```python
from build123d import *

# Parameters (mm, degrees)
SKETCH_1_R          = 2
SKETCH_1_W          = 8.7
SKETCH_1_H          = 18
EXTRUDE_1_DEPTH     = 5
FILLET_1_R          = 2
CUT_EXTRUDE_1_REACH = 58.089


with BuildPart() as part:
    # Sketch 1 → Extrude 1 (new body)
    # profile 1 of 3: a face of its own
    with BuildSketch(Plane.XY):
        with BuildLine():
            Line((39, 40), (-39, 40))
            Line((-39, 40), (-39, 0))
            Line((-39, 0), (-30.3, 0))
            ThreePointArc((-30.3, 0), (0, 30.3), (30.3, 0))
            Line((30.3, 0), (39, 0))
            Line((39, 0), (39, 40))
        make_face()
        with Locations((-34.65, 10)):
            Circle(SKETCH_1_R, mode=Mode.SUBTRACT)
        with Locations((34.65, 10)):
            Circle(SKETCH_1_R, mode=Mode.SUBTRACT)
    # profile 2 of 3: a face of its own
    with BuildSketch(Plane.XY):
        with Locations((-34.65, -9)):
            Rectangle(SKETCH_1_W, SKETCH_1_H)
        with Locations((-34.65, -10)):
            Circle(SKETCH_1_R, mode=Mode.SUBTRACT)
    # profile 3 of 3: a face of its own
    with BuildSketch(Plane.XY):
        with Locations((34.65, -9)):
            Rectangle(SKETCH_1_W, SKETCH_1_H)
        with Locations((34.65, -10)):
            Circle(SKETCH_1_R, mode=Mode.SUBTRACT)
    extrude(amount=EXTRUDE_1_DEPTH)

    # Fillet 1
    fillet_1_edges = [part.edges().sort_by_distance(p)[0] for p in [
        (-30.3, -18, 2.5),
        (-39, -18, 2.5),
        (-39, 40, 2.5),
        (39, 40, 2.5),
        (39, -18, 2.5),
        (30.3, -18, 2.5),
    ]]
    fillet(fillet_1_edges, radius=FILLET_1_R)

    # Sketch 2 → Cut-Extrude 1 (cut, up to next)
    with BuildSketch(Plane.XY.offset(5), mode=Mode.PRIVATE) as cut_extrude_1_sk1:
        with BuildLine():
            Line((-36.65, 10), (-36.65, 12))
            ThreePointArc((-36.65, 12), (-34.65, 14), (-32.65, 12))
            Line((-32.65, 12), (-32.65, 10))
            Line((-32.65, 10), (-36.65, 10))
        make_face()
    cut_extrude_1_tool1 = extrude(cut_extrude_1_sk1.sketch, amount=-CUT_EXTRUDE_1_REACH, mode=Mode.PRIVATE) & part.part
    # Sketch 2 → Cut-Extrude 1 (cut, up to next)
    with BuildSketch(Plane.XY.offset(5), mode=Mode.PRIVATE) as cut_extrude_1_sk2:
        with BuildLine():
            Line((-36.65, -10), (-36.65, -8))
            ThreePointArc((-36.65, -8), (-34.65, -6), (-32.65, -8))
            Line((-32.65, -8), (-32.65, -10))
            Line((-32.65, -10), (-36.65, -10))
        make_face()
    cut_extrude_1_tool2 = extrude(cut_extrude_1_sk2.sketch, amount=-CUT_EXTRUDE_1_REACH, mode=Mode.PRIVATE) & part.part
    cut_extrude_1_1 = cut_extrude_1_tool1.solids().sort_by_distance((-34.65, 11.8133, 5))[0]
    add(cut_extrude_1_1, mode=Mode.SUBTRACT)
    cut_extrude_1_2 = cut_extrude_1_tool2.solids().sort_by_distance((-34.65, -8.1867, 5))[0]
    add(cut_extrude_1_2, mode=Mode.SUBTRACT)
    cut_extrude_1 = cut_extrude_1_1 + cut_extrude_1_2  # Cut-Extrude 1 as one shape, for the pattern or mirror that repeats it

    # Mirror 1: Cut-Extrude 1 across plane
    add(cut_extrude_1.mirror(Plane(origin=(0, 0, 0), x_dir=(0, 0, 1), z_dir=(1, 0, 0))), mode=Mode.SUBTRACT)


solid = part.part
```
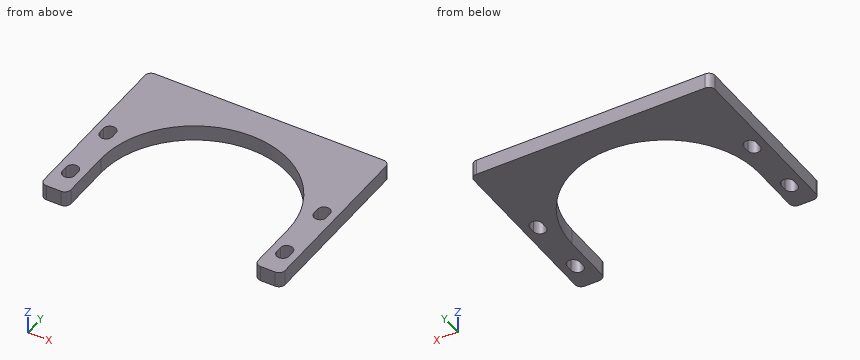
For this review, take the finished solid that the model builds, in its own axes (mm). Round coordinates to 2 decimals unless told otherwise and drop trailing zeros. Write each loop counter-clockwise with the first axis right and the second up, starting at its lowest first coordinate (ties: lowest second). Pieces come first, ordered by that corner, then holes. Notation, with made-up numbers: (80, 33) - (97, 33) arc R30 cw to (97, 59) - close; hole circle Ø7 at (-29, -7). An arc over 180 degrees is marked (long way). Write each question's results on one line, items separated by ' | '.
Item 1: Take a section at D-D on y = -11. State the section outline as (x, z) points, then the cut area to 3 significant figures.
Calculated:
outline: (-39, 0) - (-36.38, 0) - (-36.38, 5) - (-39, 5) - close; (-32.92, 0) - (-30.3, 0) - (-30.3, 5) - (-32.92, 5) - close; (30.3, 0) - (32.92, 0) - (32.92, 5) - (30.3, 5) - close; (36.38, 0) - (39, 0) - (39, 5) - (36.38, 5) - close | area: 52.4 mm^2
Item 2: To check wall thickness, follow line 1 along X through (y, z) = (-9.5, 2.25); line 2 along X through (y, z) = (-3, 0.9); line 3 along Y through (x, z) = (34, 4.5). State the ranges of each line that lie inside material, in increasing order. Write a range as from..to.
Calculated:
line 1: x = -39..-36.65, -32.65..-30.3, 30.3..32.65, 36.65..39 | line 2: x = -39..-30.3, 30.3..39 | line 3: y = -18..-11.89, -6.11..8.11, 13.89..40
Item 3: Take a section at C-C on y = 6.5. State the section outline as (x, z) points.
Calculated:
outline: (-39, 0) - (-29.59, 0) - (-29.59, 5) - (-39, 5) - close; (29.59, 0) - (39, 0) - (39, 5) - (29.59, 5) - close
Item 4: Take a section at A-A on z = 3.35. Count the separate pieces of the cut face and the enclosed holes in it, then the cut area to 3 significant figures.
Calculated:
separate pieces: 1 | enclosed holes: 4 | area: 1,900 mm^2
Item 5: Take a section at B-B on x = -34.65. State the section outline as (y, z) points, then the cut area to 3 significant figures.
Calculated:
outline: (-18, 0) - (-12, 0) - (-12, 5) - (-18, 5) - close; (-6, 0) - (8, 0) - (8, 5) - (-6, 5) - close; (14, 0) - (40, 0) - (40, 5) - (14, 5) - close | area: 230 mm^2
